Autodesk Inventor part; units mm, degrees
ref_plane "YZ Plane" through (0, 0, 0) normal (1, 0, 0) x (0, 1, 0)
ref_plane "XZ Plane" through (0, 0, 0) normal (0, 1, 0) x (-1, 0, 0)
ref_plane "XY Plane" through (0, 0, 0) normal (0, 0, 1) x (1, 0, 0)
sketch "Sketch1" plane through (0, 0, 0) normal (0, 1, 0) x (-1, 0, 0)
  line L0 (0, 0) -> (0, -51.5938)
  line L1 (0, -51.5938) -> (7.1438, -51.5938)
  line L2 (7.1438, -42.0688) -> (8.7312, -42.0688)
  line L3 (8.7312, -42.0688) -> (8.7312, -35.9728)
  line L4 (8.7312, -35.9728) -> (7.1437, -35.9728)
  line L5 (7.1438, -51.5938) -> (7.1438, -42.0688)
  line L6 (7.1437, -35.9728) -> (7.1437, -26.1938)
  line L7 (0, 0) -> (7.1437, 0)
  line L8 (7.1438, -20.6375) -> (3.9688, -20.6375)
  line L9 (3.9688, -20.6375) -> (3.9688, -23.0188)
  line L10 (3.9688, -23.0188) -> (7.1437, -26.1938)
  line L11 (7.1438, -12.446) -> (8.5408, -12.446)
  line L12 (8.5408, -12.446) -> (8.5408, -6.35)
  line L13 (8.5408, -6.35) -> (7.1438, -6.35)
  line L14 (7.1437, 0) -> (7.1438, -6.35)
  line L15 (7.1438, -12.446) -> (7.1438, -20.6375)
  dimension "d2" = 51.5938
  dimension "d3" = 7.1437
  dimension "d36" = 7.1437
  dimension "d42" = 2.3813
  dimension "d43" = 1.397
  dimension "d44" = 1.397
  dimension "d45" = 6.096
  dimension "d64" = 6.35
  dimension "d65" = 9.525
  dimension "d66" = 6.096
  dimension "d67" = 1.5875
  dimension "d68" = 9.779
  dimension "d69" = 3.9688
  dimension "d71" = 20.6375
extrude "Extrusion1" add sketch "Sketch1" along normal blind 50.292
sketch "Sketch3" plane through (-8.7312, 0, -42.0688) normal (-1, 0, 0) x (0, 0, 1)
  line L0 (6.096, 0) -> (6.096, 50.292)
  line L1 (0, 50.292) -> (6.096, 50.292)
  line L2 (0, 0) -> (6.096, 0)
  line L3 (35.7188, 0) -> (35.7188, 50.292)
  point P0 (42.0688, 0)
  point P1 (3.048, 39.1795)
  point P2 (3.048, 11.1125)
  point P3 (32.6708, 39.1795)
  point P4 (32.6708, 11.1125)
  dimension "d49" = 3.048
  dimension "d50" = 3.048
  dimension "d51" = 11.1125
  dimension "d52" = 11.1125
  dimension "d60" = 3.048
  dimension "d61" = 3.048
  dimension "d62" = 0
  dimension "d63" = 0
hole "Hole2" at (-8.7312, 39.1795, -39.0208) at (-8.7312, 11.1125, -39.0208) at (-8.7312, 39.1795, -9.398) at (-8.7312, 11.1125, -9.398) direction (1, 0, 0) diameter 6.35 end through all
equation "\"d36\" = d3"
equation "\"d43\" = d14"
equation "\"d44\" = d14"
equation "\"d45\" = d15"
properties part number "80-20 extrusion rail"
The model under review builds one solid part; all positions refer to its coordinate system, in mm. A direction names the side the tool comes from. Give positions to 0.01 mm unless a question says otherwise; leave off trailing zeros. Loops run counter-clockwise (first coordinate to the right, second up) from the corner with the lowest first, then second, coordinate; pieces in that order, holes last. Notation, with made-up numbers: (85.25, 5.5) -> (131.25, 5.5) arc R32 cw to (131.25, 31.5) -> close; hole circle Ø2 at (-3.5, 63.25). An arc over 180 degrees is marked (long way). Put each result on its own line as item: value. Start each with the question number.
1. We need section C-C on y = 7. State the section outline as (x, z) points.
2. We need section B-B on y = 13. State the section outline as (x, z) points.
3. Clearance check with flat-ended pins moving along their axes: P1, Ø5, axis at y = 14, z = -3.5, coming from the -X side; P2, Ø0.8, axis at x = -8, y = 3, coming from the -Z side; P3, Ø4, axis at y = 11.11, z = -39.02, coming from the +X side; P4, Ø0.7, axis at x = -8, y = 6, coming from the +Z side. State where each tip first meets the part, or that it passes through.
4. We need section A-A on x = -6. State how many separate pieces and enclosed holes the cut face has, then the cut area to 3 significant figures.
5. For faces 1 (the face through (-8, 45, -42.069)), 2 (the face through (-8.731, 4, -39)), 3 (the face through (-3, 50.292, -25)), 4 (the face through (-8.541, 4, -9)), 5 (the face through (-8, 5, -35.973)), list the 3-axis set-ups (+Z, -Z, +X, -X, +Y, -Y) from which the entire face can be reached by the end or side of a thin tool; tool diameter is ignored.
6. Wall thickness on probe 1 along Z at (x, y) = (-8, 3); probe 2 along Y at (x, z) = (-2.75, -11.5); probe 3 along Z at (x, y) = (-7.25, 41.5) (3 decimals): over which ranges is each line inside the solid? List them lowest first.
7. Mouldability with a two-part tool opening along Z and no side actions: class faces 6 (the face through (-4, 25, -51.594)), 7 (the face through (-8, 45, -35.973)), 8 (the face through (-8, 45, -6.35)), 9 (the face through (-8, 5, -12.446)) as released by +Z, released by -Z, zero draft, split by the parting line, or undercut.
Determined:
1. outline: (-8.73, -42.07) -> (-7.14, -42.07) -> (-7.14, -51.59) -> (0, -51.59) -> (0, 0) -> (-7.14, 0) -> (-7.14, -6.35) -> (-8.54, -6.35) -> (-8.54, -12.45) -> (-7.14, -12.45) -> (-7.14, -20.64) -> (-3.97, -20.64) -> (-3.97, -23.02) -> (-7.14, -26.19) -> (-7.14, -35.97) -> (-8.73, -35.97) -> close
2. outline: (-8.73, -42.07) -> (-7.14, -42.07) -> (-7.14, -51.59) -> (0, -51.59) -> (0, -41.57) -> (-8.73, -41.57) -> close; (-8.73, -36.47) -> (0, -36.47) -> (0, -11.95) -> (-8.54, -11.95) -> (-8.54, -12.45) -> (-7.14, -12.45) -> (-7.14, -20.64) -> (-3.97, -20.64) -> (-3.97, -23.02) -> (-7.14, -26.19) -> (-7.14, -35.97) -> (-8.73, -35.97) -> close; (-8.54, -6.84) -> (0, -6.84) -> (0, 0) -> (-7.14, 0) -> (-7.14, -6.35) -> (-8.54, -6.35) -> close
3. P1: x = -7.14
3. P2: z = -42.07
3. P3: through
3. P4: z = -6.35
4. separate pieces: 2
4. enclosed holes: 4
4. area: 2,250 mm^2
5. face 1: -Z, -X, +Y, -Y
5. face 2: +Z, -Z, -X, +Y, -Y
5. face 3: +Z, -Z, +X, -X, +Y
5. face 4: +Z, -X, +Y, -Y
5. face 5: -X, +Y, -Y
6. probe 1: -42.07 to -35.97, -12.45 to -6.35
6. probe 2: 0 to 8.73, 13.49 to 36.8, 41.56 to 50.29
6. probe 3: -42.069 to -41.188, -36.854 to -35.973, -12.446 to -11.565, -7.231 to -6.35
7. face 6: released by -Z
7. face 7: undercut
7. face 8: released by +Z
7. face 9: undercut
